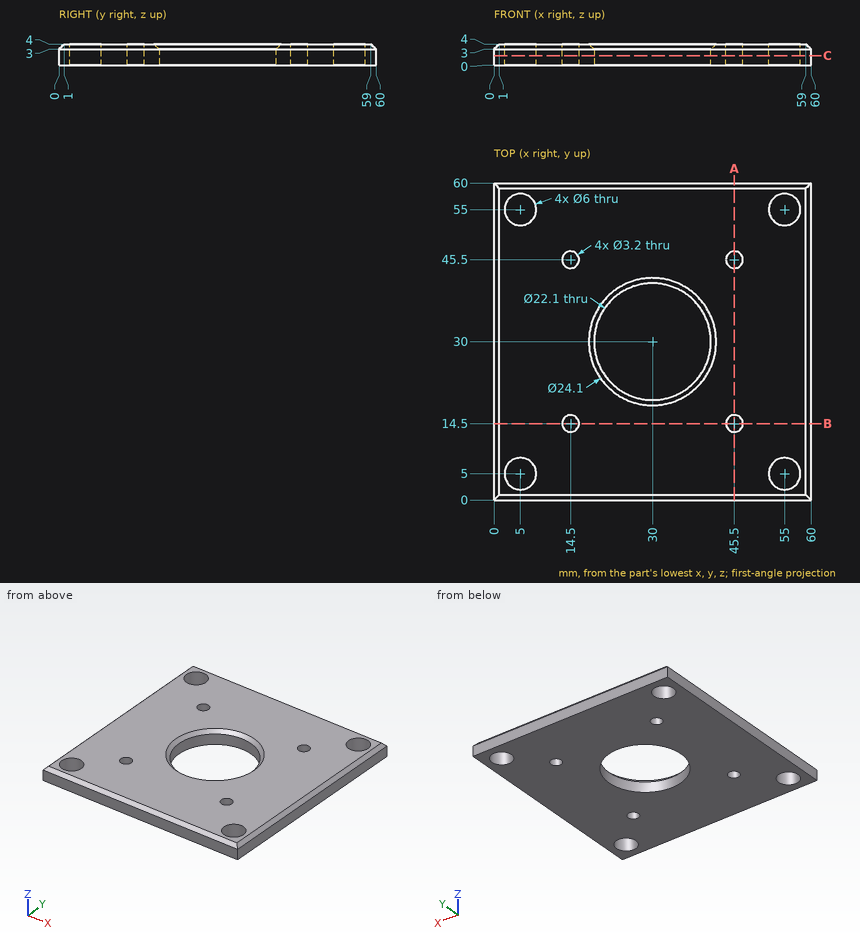
Part print with two shaded views. Sizes in mm from the minimum x, y, z corner. Coordinates: 2 decimals unless noted, no trailing zeros. Order: outer loops, then holes, each group sorted by start corner. A loop starts at its lowest first (then second) coordinate and runs counter-clockwise, first axis right, second up. Notation, with made-up numbers: M 13,58 L 48,58 A11 cw 48,69 Z; hole C 56,-21 d11. An arc over 180 degrees is marked long. Use a Markdown table: item, result.
(1) Cut at A-A on x = 45.5. Write the cut outline in (y, z).
A:
| item | result |
|---|---|
| outline | M 0,0 L 12.9,0 L 12.9,4 L 1,4 L 0,3 Z; M 16.1,0 L 43.9,0 L 43.9,4 L 16.1,4 Z; M 47.1,0 L 60,0 L 60,3 L 59,4 L 47.1,4 Z |
(2) Cut at C-C on z = 1.8. State how many separate pieces and enclosed holes the cut face has, then the cut area to 3 significant figures.
A:
| item | result |
|---|---|
| separate pieces | 1 |
| enclosed holes | 9 |
| area | 3,070 mm^2 |
(3) Probe L1, parallel to Y at x = 14.5, z = 2.9; L2, parallel to Y at x = 5, z = 1.9. List the from-to ranges inside material, lowest first.
A:
| item | result |
|---|---|
| L1 | y = 0 to 12.9, 16.1 to 43.9, 47.1 to 60 |
| L2 | y = 0 to 2, 8 to 52, 58 to 60 |
